Geometry check sheet. Reference: the model listing, model coordinates, mm. Face numbers are marked on the shaded views. A direction names the side the tool comes from. Round coordinates to 2 decimals unless told otherwise and drop trailing zeros. Order: outer loops, then holes, each group sorted by start corner. A loop starts at its lowest first (then second) coordinate and runs counter-clockwise, first axis right, second up.
(1) Cross-section at A-A on z = -5.5. Enter the section's corners in (x, y), and give its area (3 significant figures).
(2) Thickness scan on L1, parallel to X at y = 7.5, z = -13; L2, parallel to Y at x = -6, z = -7.5; L3, parallel to Y at x = -61.25, z = -9.75. Record the ranges inside material, lowest first.
(3) Gauge pin test, flat ends, axial feed: P1, Ø3.5, axis at y = 15.5, z = -9.75, coming from the -X side; P2, Ø1.1, axis at x = -7, y = -5.5, coming from the -Z side; P3, Ø0.5, axis at x = -1, z = -24.5, coming from the +Y side; P4, Ø10, axis at x = 29.5, y = -7, coming from the -Z side. Record the tip position at first contact, or that the pin passes through.
(4) Cross-section at B-B on y = 0. Enter the section's corners in (x, z).
(5) Set-up check for the marked faces 4, 5 and 6: record each of +Z, -Z, +X, -X, +Y, -Y from which the full face is reachable in a straight line by a thin tool's end or side.
(6) Cross-section at D-D on x = 18. Enter the section's corners in (y, z), and give its area (3 significant figures).
(7) Cross-section at C-C on x = 37.5. Enter the section's corners in (y, z).
(8) Draft check along X on the marked faces 1, 2 and 3. Enter one of: pulls with the +X half, pulls with the -X half, needs draft (parallel to the pull), parting line crosses it, or undercut.
Autodesk Inventor part; units mm, degrees
ref_plane "YZ Plane" through (0, 0, 0) normal (1, 0, 0) x (0, 1, 0)
ref_plane "XZ Plane" through (0, 0, 0) normal (0, 1, 0) x (-1, 0, 0)
ref_plane "XY Plane" through (0, 0, 0) normal (0, 0, 1) x (1, 0, 0)
sketch "Sketch2" plane through (0, 0, 0) normal (0, 0, 1) x (1, 0, 0)
  line L0 (-60, 21.25) -> (60, 21.25)
  line L1 (60, 21.25) -> (60, -21.25)
  line L2 (60, -21.25) -> (-60, -21.25)
  line L3 (-60, -21.25) -> (-60, 21.25)
  line L4 (-60, 21.25) -> (60, -21.25) construction
  line L5 (60, 21.25) -> (-60, -21.25) construction
  line L6 (-64, 25.5) -> (64, 25.5)
  line L7 (64, 25.5) -> (64, -25.5)
  line L8 (64, -25.5) -> (-64, -25.5)
  line L9 (-64, -25.5) -> (-64, 25.5)
  line L10 (-64, 25.5) -> (64, -25.5) construction
  line L11 (64, 25.5) -> (-64, -25.5) construction
  line L12 (-15, 12.5) -> (15, 12.5)
  line L13 (15, 12.5) -> (15, -12.5)
  line L14 (15, -12.5) -> (-15, -12.5)
  line L15 (-15, -12.5) -> (-15, 12.5)
  line L16 (-15, 12.5) -> (15, -12.5) construction
  line L17 (15, 12.5) -> (-15, -12.5) construction
  circle A0 centre (37.5, 0) radius 18
  circle A1 centre (-37.5, 0) radius 18
  point P0 (0, 0)
  point P1 (0, 0)
  dimension "d0" = 120
  dimension "d1" = 42.5
  dimension "d2" = 60
  dimension "d3" = 21.25
  dimension "d4" = 128
  dimension "d5" = 51
  dimension "d28" = 30
  dimension "d29" = 25
  dimension "d32" = 45
  dimension "d33" = 36
  dimension "d34" = 22.5
  dimension "d35" = 45
  dimension "d36" = 36
  dimension "d37" = 22.5
  dimension "d38" = 21.25
  dimension "d39" = 21.25
extrude "Extrusion1" add sketch "Sketch2" against normal blind 4 contours L0 L1 L2 L3 | L12 L13 L14 L15 | A0 | A1
extrude "Extrusion2" add sketch "Sketch2" against normal blind 20 contours L6 L7 L8 L9
fillet "Fillet1" radius 2 4 edges at (-64, 0, 0) (0, 25.5, 0) (64, 0, 0) (0, -25.5, 0)
sketch "Sketch3" plane through (-64, -25.5, -20) normal (-1, 0, 0) x (0, 0, 1)
  line L0 (16, 4.25) -> (16, 46.75)
  line L1 (16, 4.25) -> (-26.5, 4.25)
  line L2 (-26.5, 4.25) -> (-26.5, 46.75)
  line L3 (-26.5, 46.75) -> (16, 46.75)
  line L4 (16, 46.75) -> (16, 4.25)
  circle A0 centre (-5.25, 25.5) radius 11 construction
  circle A1 centre (-5.25, 25.5) radius 12.5
  circle A2 centre (10.25, 10) radius 1.5
  circle A3 centre (10.25, 41) radius 1.5
  point P0 (20, 25.5)
  dimension "d11" = 42.5
  dimension "d12" = 22
  dimension "d13" = 25
  dimension "d16" = 3
  dimension "d17" = 3
  dimension "d19" = 15.5
  dimension "d20" = 21.25
  dimension "d21" = 42.5
  dimension "d22" = 21.25
  dimension "d23" = 15.5
  dimension "d24" = 15.5
  dimension "d25" = 15.5
extrude "Extrusion3" cut sketch "Sketch3" against normal blind 150 contours A1
sketch "Sketch5" plane through (-64, 25.5, -20) normal (0, 1, 0) x (1, 0, 0)
  point P0 (64, -20)
extrude "Extrusion4" cut sketch "Sketch3" against normal blind 150 contours A2 | A3
extrude "Extrusion5" add sketch "Sketch2" against normal blind 24 contours L12 L13 L14 L15
extrude "Extrusion6" cut sketch "Sketch2" against normal blind 24 contours A0 | A1
sketch "Sketch6" plane through (0, 0, -24) normal (0, 0, -1) x (-1, 0, 0)
  line L0 (-10.3, 8) -> (10.3, 8)
  line L1 (10.3, 8) -> (10.3, -8)
  line L2 (10.3, -8) -> (-10.3, -8)
  line L3 (-10.3, -8) -> (-10.3, 8)
  line L4 (-10.3, 8) -> (10.3, -8) construction
  line L5 (10.3, 8) -> (-10.3, -8) construction
  line L6 (-15, -12.5) -> (-15, 12.5)
  line L7 (15, -12.5) -> (-15, -12.5)
  line L8 (-15, 12.5) -> (15, 12.5)
  line L9 (15, 12.5) -> (15, -12.5)
  line L10 (15, -12.5) -> (-15, -12.5)
  line L11 (-15, -12.5) -> (-15, 12.5)
  line L12 (15, 12.5) -> (15, -12.5)
  line L13 (-15, 12.5) -> (15, 12.5)
  line L14 (15, 12.5) -> (15, 4.5)
  line L15 (15, 4.5) -> (-15, 4.5)
  line L16 (-15, 4.5) -> (-15, 12.5)
  point P0 (0, 0)
  dimension "d42" = 20.6
  dimension "d43" = 16
  dimension "d46" = 12.5
extrude "Extrusion7" add sketch "Sketch6" along normal blind 1 contours L3 L15 L6 L8 L9 L1 L0 | L3 L2 L1 L15 L9 L7 L6
extrude "Extrusion8" cut sketch "Sketch6" along normal mid plane 5 contours L3 L15 L6 L8 L9 L1 L0 | L0 L1 L15 L3
sketch "Sketch7" plane through (0, 0, -24) normal (0, 0, -1) x (-1, 0, 0)
  line L0 (10.3, -8) -> (-10.3, -8)
  line L1 (10.3, 4.5) -> (-10.3, 4.5)
  line L2 (10.3, -8) -> (-10.3, -8)
  line L3 (-10.3, -8) -> (-10.3, 4.5)
  line L4 (-10.3, 4.5) -> (10.3, 4.5)
  line L5 (10.3, 4.5) -> (10.3, -8)
  circle A0 centre (7.3, -5.55) radius 0.5
  circle A1 centre (-7.3, -5.55) radius 0.5
  point P0 (0, 0)
  dimension "d49" = 1
  dimension "d50" = 1
  dimension "d51" = 3
  dimension "d52" = 3
  dimension "d53" = 2.45
  dimension "d54" = 2.45
  dimension "d55" = 14.6
extrude "Extrusion9" cut sketch "Sketch7" against normal blind 5 contours A0 | A1
sketch "Sketch8" plane through (-64, -25.5, -2) normal (-1, 0, 0) x (0, 0, 1)
  circle A0 centre (-7.75, 10) radius 1.5
  circle A1 centre (-7.75, 10) radius 3
  circle A2 centre (-7.75, 41) radius 1.5
  circle A3 centre (-7.75, 41) radius 3
  point P0 (2, 25.5)
  dimension "d58" = 6
  dimension "d59" = 6
extrude "Extrusion10" cut sketch "Sketch8" against normal blind 1
sketch "Sketch9" plane through (64, -25.5, -2) normal (1, 0, 0) x (0, 0, -1)
  circle A0 centre (7.75, 41) radius 1.5
  circle A1 centre (7.75, 41) radius 3
  circle A2 centre (7.75, 10) radius 1.5
  circle A3 centre (7.75, 10) radius 3
  point P0 (-2, 25.5)
  dimension "d62" = 6
  dimension "d63" = 6
extrude "Extrusion11" cut sketch "Sketch9" against normal blind 1
equation "\"d34\" = 0.5 * d32"
equation "\"d37\" = 0.5 * d35"
equation "\"d38\" = 0.5 * d1"
equation "\"d39\" = 0.5 * d1"
equation "\"d20\" = 0.5 * d21"
equation "\"d21\" = d11"
equation "\"d22\" = 0.5 * d11"
equation "\"d52\" = d51"
equation "\"d54\" = d53"
properties part number "Baseplate"
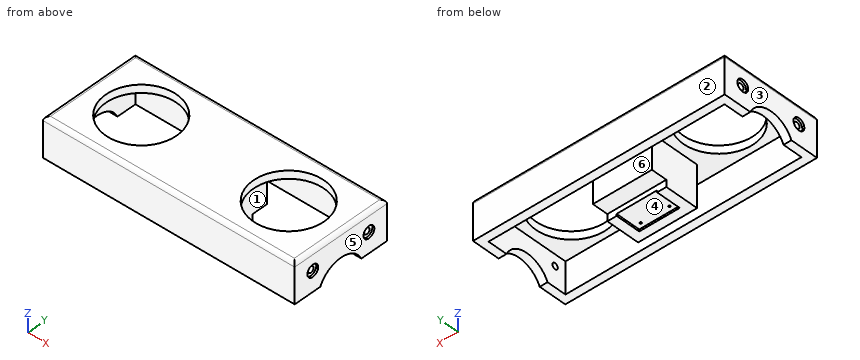
Found:
1. outline: (-64, -25.5) - (64, -25.5) - (64, 25.5) - (-64, 25.5) - close; (-15, -12.5) - (15, -12.5) - (15, 12.5) - (-15, 12.5) - close; hole (-60, -21.25) - (60, -21.25) - (60, 21.25) - (-60, 21.25) - close
1. area: 2,180 mm2
2. L1: x = -64 to -60, -15 to 15, 60 to 64
2. L2: y = -25.5 to -21.25, -12.5 to 12.5, 21.25 to 25.5
2. L3: y = -25.5 to -17, -14 to 14, 17 to 25.5
3. P1: stops at x = -63
3. P2: stops at z = -24
3. P3: stops at y = -8
3. P4: passes through
4. outline: (-64, -12.75) - (-60, -12.75) - (-60, -4) - (-55.5, -4) - (-55.5, 0) - (-62, 0) arc R2 ccw to (-64, -2) - close; (-19.5, -4) - (-15, -4) - (-15, -25) - (-10.3, -25) - (-10.3, -24) - (10.3, -24) - (10.3, -25) - (15, -25) - (15, -4) - (19.5, -4) - (19.5, 0) - (-19.5, 0) - close; (55.5, -4) - (60, -4) - (60, -12.75) - (64, -12.75) - (64, -2) arc R2 ccw to (62, 0) - (55.5, 0) - close
5. face 4: -Z, +Y
5. face 5: +Z, -Z, +X, +Y, -Y
5. face 6: -Z
6. outline: (-25.5, -20) - (-21.25, -20) - (-21.25, -4) - (21.25, -4) - (21.25, -20) - (25.5, -20) - (25.5, -2) arc R2 ccw to (23.5, 0) - (-23.5, 0) arc R2 ccw to (-25.5, -2) - close
6. area: 338 mm2
7. outline: (-25.5, -20) - (-21.25, -20) - (-21.25, -4) - (-18, -4) - (-18, 0) - (-23.5, 0) arc R2 ccw to (-25.5, -2) - close; (18, -4) - (21.25, -4) - (21.25, -20) - (25.5, -20) - (25.5, -2) arc R2 ccw to (23.5, 0) - (18, 0) - close
8. face 1: undercut
8. face 2: needs draft
8. face 3: pulls with the -X half
